Work out the finished part from the listing and answer in its coordinate system (mm). Coordinates: 2 decimals unless noted, no trailing zeros. Order: outer loops, then holes, each group sorted by start corner. A loop starts at its lowest first (then second) coordinate and runs counter-clockwise, first axis right, second up. Notation, with made-up numbers: M 13,34 L 69,34 A25 cw 69,48 Z; hole C -0.5,34.5 d5. An arc over 180 degrees is marked long. Write item = value, one per line. Start each with the question number.
Q1. Find section A-A on x = 0. Give the vertices of the cut face in (y, z), and give its area (3 significant figures).
Q2. Straight lines are drawn through the part: line 1 along X through (y, z) = (37.5, 0); line 2 along X through (y, z) = (66, -2.5); line 3 along X through (y, z) = (71, 3.75). For each, find the intervals that lie inside material, in ascending order.
Q3. Each of these flat-tipped pins is pushed along its axis until it touches: P1, Ø2, axis at y = 45.5, z = -3, coming from the +X side; P2, Ø1, axis at x = 3, z = 5, coming from the -Y side; P3, Ø1, axis at y = 67, z = -3, coming from the +X side; P4, Ø1.5, axis at x = 5.5, y = 43, coming from the -Z side. Where does it stop, or does it pass through?
Q4. Find section C-C on z = -0.75. Give the vertices of the cut face in (x, y).
```python
from build123d import *

# Parameters (mm, degrees)
SKETCH1_R           = 2.9337
BOSS_EXTRUDE1_DEPTH = 76.2


with BuildPart() as part:
    # Sketch1 → Boss-Extrude1 (new body)
    with BuildSketch(Plane(origin=(0, 0, 0), x_dir=(1, 0, 0), z_dir=(0, 1, 0))):
        with BuildLine():
            Line((-4.70551159, -4.549815043), (-3.666174521, -6.349999904))
            Line((-3.666174521, -6.349999904), (-1.587501539, -6.349999904))
            ThreePointArc((-1.587501539, -6.349999904), (-3.85e-07, -4.76249875), (1.587501539, -6.349999904))
            Line((1.587501539, -6.349999904), (3.666173825, -6.349999904))
            Line((3.666173825, -6.349999904), (4.705510929, -4.549815232))
            ThreePointArc((4.705510929, -4.549815232), (4.124445601, -2.381249904), (6.293010929, -1.800184575))
            Line((6.293010929, -1.800184575), (7.332348034, 9.6e-08))
            Line((7.332348034, 9.6e-08), (6.293011178, 1.800184715))
            ThreePointArc((6.293011178, 1.800184715), (4.124445902, 2.381250241), (4.705511428, 4.549815516))
            Line((4.705511428, 4.549815516), (3.666174521, 6.350000222))
            Line((3.666174521, 6.350000222), (1.587498461, 6.350000222))
            ThreePointArc((1.587498461, 6.350000222), (3.85e-07, 4.762502146), (-1.587498461, 6.350000222))
            Line((-1.587498461, 6.350000222), (-3.666173825, 6.350000222))
            Line((-3.666173825, 6.350000222), (-4.705511038, 4.549815614))
            ThreePointArc((-4.705511038, 4.549815614), (-4.124445841, 2.38125025), (-6.293011205, 1.800185053))
            Line((-6.293011205, 1.800185053), (-7.332348419, 4.44e-07))
            Line((-7.332348419, 4.44e-07), (-6.293011423, -1.80018429))
            ThreePointArc((-6.293011423, -1.80018429), (-4.12444613, -2.38124975), (-4.70551159, -4.549815043))
        make_face()
        with Locations(Location((0, 0, 0), (0, 0, 90))):
            Circle(SKETCH1_R, mode=Mode.SUBTRACT)
    extrude(amount=BOSS_EXTRUDE1_DEPTH)


solid = part.part
```
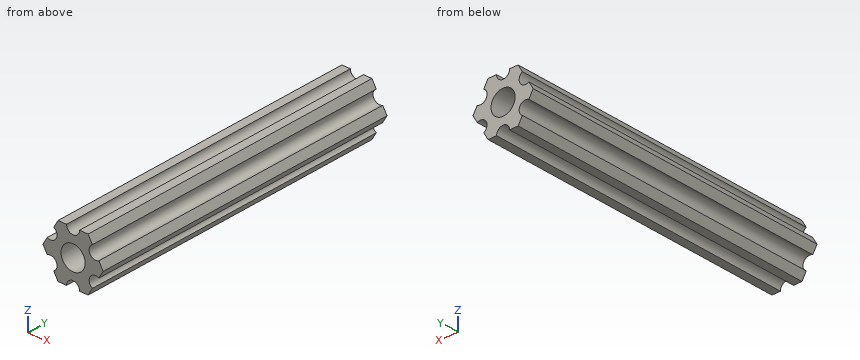
Findings below:
q1.outline = M 0,-4.76 L 76.2,-4.76 L 76.2,-2.93 L 0,-2.93 Z; M 0,2.93 L 76.2,2.93 L 76.2,4.76 L 0,4.76 Z
q1.area = 279 mm^2
q2.line_1 = -7.33 to -2.93, 2.93 to 7.33
q2.line_2 = -4.06 to -1.54, 1.54 to 4.06
q2.line_3 = -4.02 to 4.02
q3.P1 = 4.43
q3.P2 = 0
q3.P3 = 4.06
q3.P4 = -1.78
q4.outline = M -6.9,0 L -2.84,0 L -2.84,76.2 L -6.9,76.2 Z; M 2.84,0 L 6.9,0 L 6.9,76.2 L 2.84,76.2 Z
